Work out the finished part from the listing and answer in its coordinate system (mm). A direction names the side the tool comes from. Round coordinates to 2 decimals unless told otherwise and drop trailing zeros. Write each loop counter-clockwise with the first axis right and the second up, starting at its lowest first coordinate (ties: lowest second). Pieces come first, ordered by that corner, then holes. Notation, with made-up numbers: (-16, 11) -> (38, 11) arc R25 ccw to (38, 39) -> close; hole circle Ø10 at (41.5, -17.75). An arc over 180 degrees is marked (long way). One line per question, with ' | ' between items. Start each with the question number.
```python
from build123d import *

# Parameters (mm, degrees)
SKETCH1_W           = 100
SKETCH1_H           = 20
SKETCH1_R           = 5
BOSS_EXTRUDE1_DEPTH = 30
SKETCH4_W           = 20
SKETCH4_H           = 20
CUT_EXTRUDE1_DEPTH  = 25
BOSS_EXTRUDE2_REACH = 108.301
SKETCH5_R           = 5


with BuildPart() as part:
    # Sketch1 → Boss-Extrude1 (new body)
    with BuildSketch(Plane.XY):
        with Locations((50, 10)):
            Rectangle(SKETCH1_W, SKETCH1_H)
        with Locations((90, 10)):
            Circle(SKETCH1_R, mode=Mode.SUBTRACT)
    extrude(amount=BOSS_EXTRUDE1_DEPTH)

    # Sketch4 → Cut-Extrude1 (cut)
    with BuildSketch(Plane.ZY):
        with Locations((15, 10)):
            Rectangle(SKETCH4_W, SKETCH4_H)
    extrude(amount=-CUT_EXTRUDE1_DEPTH, mode=Mode.SUBTRACT)

    # Sketch5 → Boss-Extrude2 (add, up to next)
    with BuildSketch(Plane.XY.offset(30), mode=Mode.PRIVATE) as boss_extrude2_sk1:
        with Locations(Location((10, 10, 0), (0, 0, 270))):
            Circle(SKETCH5_R)
    boss_extrude2_tool1 = extrude(boss_extrude2_sk1.sketch, amount=-BOSS_EXTRUDE2_REACH, mode=Mode.PRIVATE) - part.part
    add(boss_extrude2_tool1.solids().sort_by_distance((10, 10, 30))[0])


solid = part.part
```
(1) For faces 4 (the cylindrical face through (11.5, 5.23, 15.14)), 5 (the cylindrical face through (94.619, 8.085, 14.79)), determine the directions among +Z, -Z, +X, -X, +Y, -Y from which every point of the face is accessible in a straight line to the end or side of a thin tool.
(2) Consider L1, parallel to Y at x = 90, z = 13.25; L2, parallel to X at y = 6.25, z = 18.5; L3, parallel to X at y = 5.75, z = 5.25. Determine where each line is inside the solid, lowest interval first.
(3) A cutting plane is placed at A-A, the plane y = 10. Determine the outline of the cut face in (x, z), then the cut area to 3 significant figures.
(4) The mould has two halves that part along X. Classify faces 1 (the flat face through (60, 20, 15)), 2 (the flat face through (25, 10, 15)), 3 (the flat face through (0, 10, 27)): +X half, -X half, draft (parallel to the pull), parting line (faces both ways), or undercut.
(5) A cutting plane is placed at D-D, the plane x = 10. Determine the outline of the cut face in (y, z), then the cut area to 3 significant figures.
(6) A cutting plane is placed at B-B, the plane x = 20. Determine the outline of the cut face in (y, z), then the cut area to 3 significant figures.
(7) Given pin 1 Ø3 at (y, z) = (12, 11) entering from -X, flat-ended and moving along its own axis, determine where the tip first touches the part or whether it passes through.
(8) A cutting plane is placed at C-C, the plane z = 11.25. Determine the outline of the cut face in (x, y), then the cut area to 3 significant figures.
Returned:
1) face 4: none | face 5: +Z, -Z
2) L1: 0 to 5, 15 to 20 | L2: 6.69 to 13.31, 25 to 86.69, 93.31 to 100 | L3: 7.37 to 12.63, 25 to 87.37, 92.63 to 100
3) outline: (0, 0) -> (85, 0) -> (85, 30) -> (0, 30) -> (0, 25) -> (5, 25) -> (5, 5) -> (0, 5) -> close; (95, 0) -> (100, 0) -> (100, 30) -> (95, 30) -> close; hole (15, 5) -> (25, 5) -> (25, 25) -> (15, 25) -> close | area: 2,400 mm2
4) face 1: draft | face 2: undercut | face 3: -X half
5) outline: (0, 0) -> (20, 0) -> (20, 5) -> (15, 5) -> (15, 25) -> (20, 25) -> (20, 30) -> (0, 30) -> (0, 25) -> (5, 25) -> (5, 5) -> (0, 5) -> close | area: 400 mm2
6) outline: (0, 0) -> (20, 0) -> (20, 5) -> (0, 5) -> close; (0, 25) -> (20, 25) -> (20, 30) -> (0, 30) -> close | area: 200 mm2
7) pin 1: x = 5.03
8) outline: circle Ø10 at (10, 10); (25, 0) -> (100, 0) -> (100, 20) -> (25, 20) -> close; hole circle Ø10 at (90, 10) | area: 1,500 mm2
